Geometry check sheet. Reference: the model listing, model coordinates, mm. Face numbers are marked on the shaded views. Give positions to 0.01 mm unless a question says otherwise; leave off trailing zeros. Loops run counter-clockwise (first coordinate to the right, second up) from the corner with the lowest first, then second, coordinate; pieces in that order, holes last. Notation, with made-up numbers: (13, -30.5) -> (21, -30.5) arc R30 cw to (21, -0.5) -> close; hole circle Ø6 at (-3.75, -25). An arc over 180 degrees is marked (long way). Answer in a Markdown table with one row per item. Add a question column.
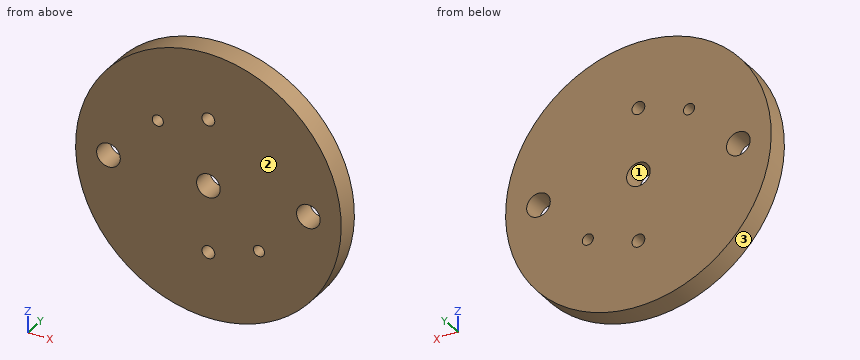
```python
from build123d import *

# Parameters (mm, degrees)
SKETCH1_R                    = 37.973
BOSS_EXTRUDE1_DEPTH          = 3.175
H_0_266_DIAMETER_HOLE1_D     = 6.7564
F_27_0_144_DIAMETER_HOLE1_D  = 3.6576
F_1_8_0_125_DIAMETER_HOLE1_D = 3.175
H_0_266_DIAMETER_HOLE2_D     = 6.7564


with BuildPart() as part:
    # Sketch1 → Boss-Extrude1 (new, symmetric)
    with BuildSketch(Plane(origin=(0, 0, 0), x_dir=(1, 0, 0), z_dir=(0, 1, 0))):
        with Locations(Location((0, 0, 0), (0, 0, 270))):
            Circle(SKETCH1_R)
    extrude(amount=BOSS_EXTRUDE1_DEPTH, both=True)

    # H (0.266) Diameter Hole1 (through all)
    with Locations(Plane(origin=(0, 3.175, 0), x_dir=(1, 0, 0), z_dir=(0, 1, 0))):
        with Locations((-28.575, 0), (28.575, 0)):
            Hole(H_0_266_DIAMETER_HOLE1_D / 2)

    # #27 (0.144) Diameter Hole1 (through all)
    with Locations(Plane(origin=(0, 3.175, 0), x_dir=(1, 0, 0), z_dir=(0, 1, 0))):
        with Locations((0, 19.05), (0, -19.05)):
            Hole(F_27_0_144_DIAMETER_HOLE1_D / 2)

    # 1/8 (0.125) Diameter Hole1 (through all)
    with Locations(Plane(origin=(0, 3.175, 0), x_dir=(1, 0, 0), z_dir=(0, 1, 0))):
        with Locations((14.469766177, 14.266333333), (-14.469766177, -14.266333333)):
            Hole(F_1_8_0_125_DIAMETER_HOLE1_D / 2)

    # H (0.266) Diameter Hole2 (through all)
    with Locations(Plane(origin=(0, 3.175, 0), x_dir=(1, 0, 0), z_dir=(0, 1, 0))):
        with Locations((0, 0)):
            Hole(H_0_266_DIAMETER_HOLE2_D / 2)


solid = part.part
```
1. Release check for a two-part mould opening along X. For the marked faces 1, 2 and 3 record: released by +X, released by -X, zero draft, split by the parting line, or undercut.
2. Sectioned sample at C-C (z = -19.05). Enter the section's corners in (x, y) (3 decimals).
3. Sectioned sample at B-B (x = -31). Enter the section's corners in (y, z) (3 decimals), plus the area to 3 significant figures.
4. Sectioned sample at D-D (y = 1). Count the separate pieces of the cut face and the enclosed holes in it, plus the area to 3 significant figures.
5. Sectioned sample at A-A (z = 0). Enter the section's corners in (x, y) (3 decimals), plus the area to 3 significant figures.
6. Material ranges on L1, parallel to X at y = -0.5, z = -19.05; L2, parallel to Z at x = -13.5, y = 1; L3, parallel to Z at x = 28.5, y = 1, recorded low to high. Write a range as from..to.
7. Gauge pin test, flat ends, axial feed: pin 1 Ø1.5 at (y, z) = (0.5, -3.5) entering from +X; pin 2 Ø9 at (x, z) = (-28.575, 0) entering from +Y (3 decimals); pin 3 Ø2 at (x, y) = (14.5, 1.5) entering from -Z. Record the tip position at first contact, or that the pin passes through.
Response:
| question | item | result |
|---|---|---|
| 1 | face 1 | undercut |
| 1 | face 2 | zero draft |
| 1 | face 3 | split by the parting line |
| 2 | outline | (-32.849, -3.175) -> (-1.829, -3.175) -> (-1.829, 3.175) -> (-32.849, 3.175) -> close; (1.829, -3.175) -> (32.849, -3.175) -> (32.849, 3.175) -> (1.829, 3.175) -> close |
| 3 | outline | (-3.175, -21.931) -> (3.175, -21.931) -> (3.175, -2.352) -> (-3.175, -2.352) -> close; (-3.175, 2.352) -> (3.175, 2.352) -> (3.175, 21.931) -> (-3.175, 21.931) -> close |
| 3 | area | 249 mm2 |
| 4 | separate pieces | 1 |
| 4 | enclosed holes | 7 |
| 4 | area | 4,390 mm2 |
| 5 | outline | (-37.973, -3.175) -> (-31.953, -3.175) -> (-31.953, 3.175) -> (-37.973, 3.175) -> close; (-25.197, -3.175) -> (-3.378, -3.175) -> (-3.378, 3.175) -> (-25.197, 3.175) -> close; (3.378, -3.175) -> (25.197, -3.175) -> (25.197, 3.175) -> (3.378, 3.175) -> close; (31.953, -3.175) -> (37.973, -3.175) -> (37.973, 3.175) -> (31.953, 3.175) -> close |
| 5 | area | 354 mm2 |
| 6 | L1 | x = -32.85..-1.83, 1.83..32.85 |
| 6 | L2 | z = -35.49..13.01, 15.52..35.49 |
| 6 | L3 | z = -25.09..-3.38, 3.38..25.09 |
| 7 | pin 1 | stops at x = 37.87 |
| 7 | pin 2 | stops at y = 3.175 |
| 7 | pin 3 | stops at z = -35.49 |
